Part model, mm, in its own coordinate system. A direction names the side the tool comes from. Coordinates: 2 decimals unless noted, no trailing zeros. Loops run counter-clockwise (first coordinate to the right, second up) from the corner with the lowest first, then second, coordinate; pieces in that order, holes last. Notation, with made-up numbers: (-17, 38) -> (-3, 38) arc R21 ccw to (-3, 72) -> close; hole circle Ø3 at (11.5, -17). An arc over 180 degrees is marked (long way). One line per item, written item: value. Start each with the question number.
from build123d import *

# Parameters (mm, degrees)
SKETCH1_R               = 7.5565
BOSS_EXTRUDE1_DEPTH     = 13.97
SKETCH2_R               = 7.5565
SKETCH2_R_2             = 3.3
BOSS_EXTRUDE2_DEPTH     = 0.635
SKETCH4_R               = 8.255
SKETCH4_R_2             = 7.5565
BOSS_EXTRUDE3_DEPTH     = 9.8425
SKETCH3_W               = 2.140633032
SKETCH3_H               = 3.81
SKETCH3_W_2             = 2.256055482
CUT_EXTRUDE1_DEPTH      = 9.255
CUT_EXTRUDE1_DEPTH_BACK = 9.255


with BuildPart() as part:
    # Sketch1 → Boss-Extrude1 (new body)
    with BuildSketch(Plane(origin=(0, 0, 0), x_dir=(1, 0, 0), z_dir=(0, 1, 0))):
        Circle(SKETCH1_R)
        Polygon((-2.915618859, 5.05), (-5.831237719, 0), (-2.915618859, -5.05), (2.915618859, -5.05), (5.831237719, 0), (2.915618859, 5.05), align=None, mode=Mode.SUBTRACT)
    extrude(amount=BOSS_EXTRUDE1_DEPTH)

    # Sketch2 → Boss-Extrude2 (add)
    with BuildSketch(Plane.XZ):
        Circle(SKETCH2_R)
        Circle(SKETCH2_R_2, mode=Mode.SUBTRACT)
    extrude(amount=BOSS_EXTRUDE2_DEPTH)

    # Sketch4 → Boss-Extrude3 (add)
    with BuildSketch(Plane.XZ.offset(0.635)):
        Circle(SKETCH4_R)
        Circle(SKETCH4_R_2, mode=Mode.SUBTRACT)
    extrude(amount=-BOSS_EXTRUDE3_DEPTH)

    # Sketch3 → Cut-Extrude1 (cut, two sides)
    with BuildSketch(Plane(origin=(0, 0, 0), x_dir=(0, 0, -1), z_dir=(1, 0, 0))) as cut_extrude1_sk:
        with Locations((-7.293316516, 7.62)):
            Rectangle(SKETCH3_W, SKETCH3_H)
        with Locations((7.351027741, 7.62)):
            Rectangle(SKETCH3_W_2, SKETCH3_H)
    extrude(amount=CUT_EXTRUDE1_DEPTH, mode=Mode.SUBTRACT)
    extrude(cut_extrude1_sk.sketch, amount=-CUT_EXTRUDE1_DEPTH_BACK, mode=Mode.SUBTRACT)


solid = part.part
1) Tool access for faces 4 (the flat face through (8, 9.208, 0)), 5 (the flat face through (4.394, 6.887, -2.49)), 6 (the flat face through (-8, 9.208, 0)), 7 (the flat face through (0, 9.525, 7)), 8 (the flat face through (0, 8, -6.223)): list every direction of +Z, -Z, +X, -X, +Y, -Y with a clear straight run to the whole face (end or side of a thin tool).
2) Slice it at C-C (z = -1.5). Give the cut face in (x, y) (1 decimal).
3) Slice it at B-B (y = 10.5). Give the cut face in (x, z), then the cut area to 3 significant figures.
4) Slice it at D-D (y = 1.5). Give the cut face in (x, z) (3 decimals), then the cut area to 3 significant figures.
5) Probe line 1 (Z direction, x = 0, y = -0.2) (3 decimals); line 2 (Y direction, x = -0.5, z = 4.75) (3 decimals); line 3 (Z direction, x = 5.25, y = 12). List the from-to ranges inside material, lowest first. Write a range as from..to.
6) Pin check, flat tips, straight feed: pin 1 Ø3 at (x, z) = (-1, 2) entering from +Y; pin 2 Ø1.1 at (x, y) = (-2, 7) entering from -Z; pin 3 Ø3 at (y, z) = (5.5, -6) entering from -X; pin 4 Ø4 at (x, z) = (0, 0) entering from +Y. Stop position of each tip, or through.
7) Pull direction X, two halves, no side cores. Call faces 1 (the flat face through (0, 9.525, -7)), 2 (the cylindrical face through (-7.55, 11.62, 0.33)), 3 (the flat face through (-4.353, 6.887, -2.56)): +X half, -X half, draft (parallel to the pull), parting line (faces both ways), or undercut.
Check sheet entries:
1. face 4: +X, +Y
1. face 5: +Y
1. face 6: -X, +Y
1. face 7: +Z, +X, -X
1. face 8: -Z, +X, -X
2. outline: (-8.1, -0.6) -> (-2.9, -0.6) -> (-2.9, 0) -> (-5, 0) -> (-5, 14) -> (-7.4, 14) -> (-7.4, 9.2) -> (-8.1, 9.2) -> close; (2.9, -0.6) -> (8.1, -0.6) -> (8.1, 9.2) -> (7.4, 9.2) -> (7.4, 14) -> (5, 14) -> (5, 0) -> (2.9, 0) -> close
3. outline: circle Ø15.11 at (0, 0); hole (-5.83, 0) -> (-2.92, -5.05) -> (2.92, -5.05) -> (5.83, 0) -> (2.92, 5.05) -> (-2.92, 5.05) -> close
3. area: 91.0 mm^2
4. outline: circle Ø16.51 at (0, 0); hole (-5.831, 0) -> (-2.916, -5.05) -> (2.916, -5.05) -> (5.831, 0) -> (2.916, 5.05) -> (-2.916, 5.05) -> close
4. area: 126 mm^2
5. line 1: z = -8.255..-3.3, 3.3..8.255
5. line 2: y = -0.635..0
5. line 3: z = -5.43..-1.01, 1.01..5.43
6. pin 1: stops at y = 0
6. pin 2: stops at z = -6.22
6. pin 3: stops at x = -6.92
6. pin 4: passes through
7. face 1: draft
7. face 2: parting line
7. face 3: undercut
